Print and shaded views of the part. All mm, measured from the part's lowest x, y and z. A direction names the side the tool comes from. Round coordinates to 2 decimals unless told otherwise and drop trailing zeros. Order: outer loops, then holes, each group sorted by start corner. A loop starts at its lowest first (then second) coordinate and runs counter-clockwise, first axis right, second up. Notation, with made-up numbers: (12.5, -34.75) -> (63.5, -34.75) arc R32 ccw to (63.5, 1.25) -> close; hole circle Ø3 at (65.25, 75). An arc over 180 degrees is marked (long way). Answer as CSV lines item,"result".
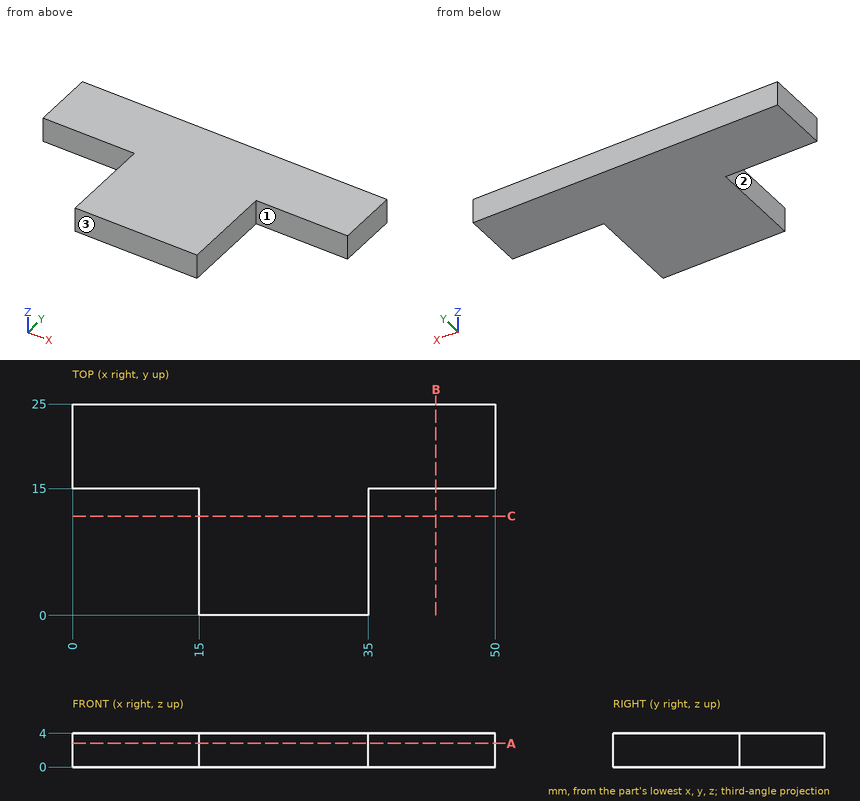
Q1. Saw through at C-C (y = 11.75). Write the cut outline in (x, z), plus the area to 3 significant figures.
Checks:
outline,"(15, 0) -> (35, 0) -> (35, 4) -> (15, 4) -> close"
area,"80.0 mm²"
Q2. Flat gauge pins, fed straight in: pin 1 (2 mm diameter, centred on x = 8.5, z = 2, fed in from -Y); pin 2 (2 mm diameter, centred on y = 9.5, z = 1.5, fed in from -X); pin 3 (1.2 mm diameter, centred on y = 9, z = 1.5, fed in from +X). Where does each tip first touch, or does it go through?
Checks:
pin 1,"y = 15"
pin 2,"x = 15"
pin 3,"x = 35"
Q3. Saw through at B-B (x = 43). Write the cut outline in (y, z), plus the area to 3 significant figures.
Checks:
outline,"(15, 0) -> (25, 0) -> (25, 4) -> (15, 4) -> close"
area,"40.0 mm²"
Q4. Saw through at A-A (z = 2.8). Write the cut outline in (x, y), plus the area to 3 significant figures.
Checks:
outline,"(0, 15) -> (15, 15) -> (15, 0) -> (35, 0) -> (35, 15) -> (50, 15) -> (50, 25) -> (0, 25) -> close"
area,"800 mm²"
Q5. Wall check: L1, parallel to X at y = 8, z = 2.8; L2, parallel to Y at x = 6, z = 1. Give the ranges that are in metal, low to high. Write a range as [from, to].
Checks:
L1,"[15, 35]"
L2,"[15, 25]"
Q6. Tool access for the marked faces 1, 2 and 3: list every direction of +Z, -Z, +X, -X, +Y, -Y with a clear straight run to the whole face (end or side of a thin tool).
Checks:
face 1,"+Z, -Z, +X, -Y"
face 2,"+Z, -Z, -X, -Y"
face 3,"+Z, -Z, +X, -X, -Y"
